```python
from build123d import *

# Parameters (mm, degrees)
SKETCH3_R           = 7.5
BOSS_EXTRUDE1_DEPTH = 8
BOSS_EXTRUDE2_DEPTH = 5
SKETCH5_W           = 56
SKETCH5_H           = 80
BOSS_EXTRUDE3_DEPTH = 5


with BuildPart() as part:
    # Sketch1 → Revolve1 (revolve)
    with BuildSketch(Plane.XY):
        Polygon((-40, 60), (0, 60), (0, 50.773502692), (-10, 40.773502692), (-10, 15.773502692), (0, 10), (0, 0), (-40, 0), (-40, 10), (-30, 15.773502692), (-30, 40.773502692), (-40, 50.773502692), align=None)
    revolve(axis=Axis((0, 0, 0), (-1, 0, 0)))

    # Sketch3 → Boss-Extrude1 (add)
    with BuildSketch(Plane(origin=(0, 0, 0), x_dir=(0, 0, -1), z_dir=(1, 0, 0))):
        Circle(SKETCH3_R)
    boss_extrude1 = extrude(amount=BOSS_EXTRUDE1_DEPTH)

    # Sketch4 → Boss-Extrude2 (add)
    with BuildSketch(Plane(origin=(8, 0, 0), x_dir=(0, 0, -1), z_dir=(1, 0, 0))):
        with BuildLine():
            Line((8.84577787, 66.773419664), (88.84577787, 66.773419664))
            Line((88.84577787, 66.773419664), (23.828381591, -18.226580336))
            ThreePointArc((23.828381591, -18.226580336), (-17.50778863, -24.361390299), (-24.872723871, 16.773419664))
            Line((-24.872723871, 16.773419664), (8.84577787, 66.773419664))
        make_face()
    boss_extrude2 = extrude(amount=-BOSS_EXTRUDE2_DEPTH)

    # Mirror1: Boss-Extrude1, Boss-Extrude2 across plane
    add(boss_extrude1.mirror(Plane(origin=(-20, 0, 0), x_dir=(0, 0, 1), z_dir=(1, 0, 0))))
    add(boss_extrude2.mirror(Plane(origin=(-20, 0, 0), x_dir=(0, 0, 1), z_dir=(1, 0, 0))))

    # Sketch5 → Boss-Extrude3 (add)
    with BuildSketch(Plane(origin=(0, 66.773419664, 0), x_dir=(1, 0, 0), z_dir=(0, 1, 0))):
        with Locations((-20, 48.84577787)):
            Rectangle(SKETCH5_W, SKETCH5_H)
    extrude(amount=-BOSS_EXTRUDE3_DEPTH)


solid = part.part
```
CAD build for the part. Positions are in the model's coordinates, mm. A direction names the side the tool comes from. Coordinates: 2 decimals unless noted, no trailing zeros. Order: outer loops, then holes, each group sorted by start corner. A loop starts at its lowest first (then second) coordinate and runs counter-clockwise, first axis right, second up. Notation, with made-up numbers: M 36.5,84 L 70.5,84 A18 cw 70.5,98 Z; hole C 36.25,85 d11. An arc over 180 degrees is marked long. Answer as CSV lines item,"result".
1) Drill centre lines: L1, parallel to X at y = -13.5, z = -20; L2, parallel to X at y = 32.5, z = -44.5; L3, parallel to X at y = 40.5, z = -58. Where is each one in solid material? Low to high. Write a range as from..to.
Verdict:
L1,"-48..-43, -30..-10, 3..8"
L2,"-48..-43, -40..0, 3..8"
L3,"-48..-43, 3..8"
2) Cut at B-B (y = 55). List the corners of the cut face in (x, z), then the cut area to 3 significant figures.
Verdict:
outline,"M -48,-79.84 L -43,-79.84 L -43,-0.91 L -48,-0.91 Z; M -40,-23.98 L 0,-23.98 L 0,23.98 L -40,23.98 Z; M 3,-79.84 L 8,-79.84 L 8,-0.91 L 3,-0.91 Z"
area,"2,710 mm2"
3) Mould opens along X. For faces 1 (the cylindrical face through (-45.54, -24.73, 16.98)), 2 (the conical face through (-0.49, -2.23, 10.04)), 3 (the flat face through (-48, 19, -17)), 4 (the flat face through (-40, 49, -14)) say: released by +X, released by -X, zero draft, split by the parting line, or undercut.
Verdict:
face 1,"zero draft"
face 2,"undercut"
face 3,"released by -X"
face 4,"undercut"
4) Cut at A-A (x = -27). List the corners of the cut face in (y, z).
Verdict:
outline,"C 0,0 d120; M 61.77,-88.85 L 66.77,-88.85 L 66.77,-8.85 L 61.77,-8.85 Z"
5) 3-axis set-ups, long thin cutter, end or side, ignore diameter. For faces 5 (the flat face through (5.54, 22.33, -54.85)), 6 (the flat face through (0, 4, -7)), 7 (the flat face through (-45.54, 22.33, -54.85)): which of +Z, -Z, +X, -X, +Y, -Y reach the whole face in a straight line?
Verdict:
face 5,"-Z, +X, -Y"
face 6,"none"
face 7,"-Z, -X, -Y"
6) Flat gauge pins, fed straight in: P1, Ø1, axis at y = -27.5, z = 29, coming from the +X side; P2, Ø2, axis at x = -17, z = -42, coming from the -Y side; P3, Ø2, axis at x = -27, y = 52.5, coming from the -Z side. Where does each tip first touch, or does it go through?
Verdict:
P1,"x = -10"
P2,"y = -43.81"
P3,"z = -30.79"
7) Cut at C-C (x = -36). List the corners of the cut face in (y, z), then the cut area to 3 significant figures.
Verdict:
outline,"C 0,0 d120; C 0,0 d24.62; M 61.77,-88.85 L 66.77,-88.85 L 66.77,-8.85 L 61.77,-8.85 Z; hole C 0,0 d93.55"
area,"5,310 mm2"
